Design review of the part built by this model. Coordinates are the model's own, in mm. Face numbers are marked on the shaded views. A direction names the side the tool comes from. Give positions to 0.01 mm unless a question says otherwise; leave off trailing zeros. Loops run counter-clockwise (first coordinate to the right, second up) from the corner with the lowest first, then second, coordinate; pieces in that order, holes last. Notation, with made-up numbers: (18.5, 12) -> (51.5, 12) arc R23 cw to (51.5, 23) -> close; hole circle Ø9 at (-23, -21.5). An arc over 180 degrees is marked (long way). Use a Markdown table: item, result. Add a question column.
1. Add section B-B (y = 16.25). State the section outline as (x, z) points.
2. To check wall thickness, follow line 1 (Y direction, x = 6.5, z = 0.3); line 2 (X direction, y = 24.25, z = 1); line 3 (Y direction, x = 8, z = 0.65). State the ranges of each line that lie inside material, in increasing order.
3. Add section C-C (z = 1.4). State the section outline as (x, y) points.
4. For the marked faces 1 and 2, list the 3-axis set-ups (+Z, -Z, +X, -X, +Y, -Y) from which the entire face can be reached by the end or side of a thin tool; tool diameter is ignored.
5. Add section A-A (x = 6.35). State the section outline as (y, z) points.
6. Draft analysis for pull direction Y (two halves, no side actions). For the marked faces 3, 4 and 5, state which applies: pulls with the +Y half, pulls with the -Y half, needs draft (parallel to the pull), parting line crosses it, or undercut.
```python
from build123d import *

# Parameters (mm, degrees)
SKETCH1_R           = 2.159
BOSS_EXTRUDE1_DEPTH = 3.2004
FILLET1_R           = 0.762


with BuildPart() as part:
    # Sketch1 → Boss-Extrude1 (new body)
    with BuildSketch(Plane.XY):
        with BuildLine():
            Line((0, 25.4), (0, 0))
            Line((0, 0), (12.7, 0))
            Line((12.7, 0), (12.7, 25.4))
            Line((12.7, 25.4), (8.8773, 25.4))
            Line((8.8773, 25.4), (8.8773, 17.4625))
            ThreePointArc((8.8773, 17.4625), (6.35, 14.9352), (3.8227, 17.4625))
            Line((3.8227, 17.4625), (3.8227, 25.4))
            Line((3.8227, 25.4), (0, 25.4))
        make_face()
        with Locations((6.35, 7.9375)):
            Circle(SKETCH1_R, mode=Mode.SUBTRACT)
    extrude(amount=BOSS_EXTRUDE1_DEPTH)

    # Fillet1
    fillet1_edges = [part.edges().sort_by_distance(p)[0] for p in [
        (3.8227, 25.4, 1.6002),
        (8.8773, 25.4, 1.6002),
        (12.7, 25.4, 1.6002),
        (12.7, 0, 1.6002),
        (0, 0, 1.6002),
        (0, 25.4, 1.6002),
    ]]
    fillet(fillet1_edges, radius=FILLET1_R)


solid = part.part
```
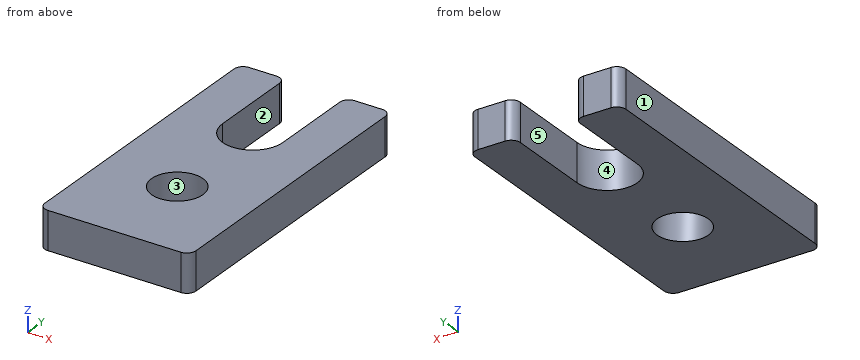
Taken from the geometry:
| question | item | result |
|---|---|---|
| 1 | outline | (0, 0) -> (4.13, 0) -> (4.13, 3.2) -> (0, 3.2) -> close; (8.57, 0) -> (12.7, 0) -> (12.7, 3.2) -> (8.57, 3.2) -> close |
| 2 | line 1 | y = 0 to 5.78, 10.09 to 14.94 |
| 2 | line 2 | x = 0 to 3.82, 8.88 to 12.7 |
| 2 | line 3 | y = 0 to 6.55, 9.33 to 15.55 |
| 3 | outline | (0, 0.76) arc R0.76 ccw to (0.76, 0) -> (11.94, 0) arc R0.76 ccw to (12.7, 0.76) -> (12.7, 24.64) arc R0.76 ccw to (11.94, 25.4) -> (9.64, 25.4) arc R0.76 ccw to (8.88, 24.64) -> (8.88, 17.46) arc R2.53 cw to (3.82, 17.46) -> (3.82, 24.64) arc R0.76 ccw to (3.06, 25.4) -> (0.76, 25.4) arc R0.76 ccw to (0, 24.64) -> close; hole circle Ø4.32 at (6.35, 7.94) |
| 4 | face 1 | +Z, -Z, -X, +Y, -Y |
| 4 | face 2 | +Z, -Z, +Y |
| 5 | outline | (0, 0) -> (5.78, 0) -> (5.78, 3.2) -> (0, 3.2) -> close; (10.1, 0) -> (14.94, 0) -> (14.94, 3.2) -> (10.1, 3.2) -> close |
| 6 | face 3 | undercut |
| 6 | face 4 | pulls with the +Y half |
| 6 | face 5 | needs draft |
